```python
from build123d import *

# Parameters (mm, degrees)
FILLET_1_R     = 1
CHAMFER_1_SIZE = 0.7


with BuildPart() as part:
    # ｽｹｯﾁ1 → 回転1 (revolve)
    with BuildSketch(Plane.XY, mode=Mode.PRIVATE) as revolve_1_sk:
        Polygon((0, 6.3), (4.5, 6.3), (4.5, 5.6), (9.5, 5.6), (9.5, 3.1), (6, 3.1), (6, 1.5), (8, 1.5), (8, 0), (3.5, 0), (3.5, 5.6), (0, 5.6), align=None)
    revolve(revolve_1_sk.sketch.rotate(Axis((0, 0, 0), (0, 1, 0)), 90), axis=Axis((0, 0, 0), (0, 1, 0)))

    # ﾌｨﾚｯﾄ1
    fillet_1_edges = [part.edges().sort_by_distance(p)[0] for p in [
        (0, 0, 8),
        (0, 5.6, 9.5),
    ]]
    fillet(fillet_1_edges, radius=FILLET_1_R)

    # 面取り1
    chamfer_1_edges = [part.edges().sort_by_distance(p)[0] for p in [
        (0, 5.6, 4.5),
    ]]
    chamfer(chamfer_1_edges, length=CHAMFER_1_SIZE - 0.0001)  # a hair under: the kernel refuses the full size


solid = part.part
```
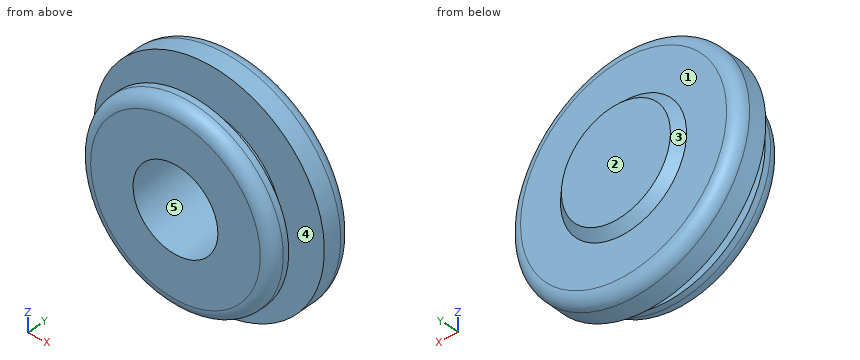
Work out the finished part from the listing and answer in its coordinate system (mm). Face numbers are marked on the shaded views. A direction names the side the tool comes from. Coordinates: 2 decimals unless noted, no trailing zeros. Loops run counter-clockwise (first coordinate to the right, second up) from the corner with the lowest first, then second, coordinate; pieces in that order, holes last.
1) Section D-D (y = 0.75) is taken. Give the vertices of the cut face in (x, z), plus the area to 3 significant figures.
Results:
outline: circle Ø15.94 at (0, 0); hole circle Ø7 at (0, 0)
area: 161 mm2
2) Section C-C (y = 3.75) is taken. Give the vertices of the cut face in (x, z).
Results:
outline: circle Ø19 at (0, 0); hole circle Ø7 at (0, 0)
3) For a pull along Y with two mould halves and no side action, classify the marked faces 3, 4 and 5 as +Y half, -Y half, draft (parallel to the pull), parting line (faces both ways), or undercut.
Results:
face 3: +Y half
face 4: undercut
face 5: draft
4) Flat-ended cylindrical pins translate along their axes: pin 1 (2 mm diameter, centred on y = 4, z = -5.5, fed in from +X); pin 2 (2 mm diameter, centred on y = 5, z = -3.5, fed in from +X). Find the tip coordinate at first contact, or state that the pin passes through.
Results:
pin 1: stops at x = 8.37
pin 2: stops at x = 9.15
5) For the marked faces 1 and 2, determine the directions among +Z, -Z, +X, -X, +Y, -Y from which every point of the face is accessible in a straight line to the end or side of a thin tool.
Results:
face 1: +Y
face 2: +Z, -Z, +X, -X, +Y
6) Consider probe 1 along Y at (x, z) = (2, 6); probe 2 along X at (y, z) = (3.5, 0); probe 3 along Y at (x, z) = (3, 7.75). Determine where each line is inside the solid, lowest interval first.
Results:
probe 1: y = 0 to 1.5, 3.1 to 5.6
probe 2: x = -9.5 to -3.5, 3.5 to 9.5
probe 3: y = 3.1 to 5.6
